from build123d import *

# Parameters (mm, degrees)
BOSS_EXTRUDE1_DEPTH = 12.7
CUT_EXTRUDE2_DEPTH  = 66.991135768
CUT_EXTRUDE1_DEPTH  = 43.597094971
FILLET1_R           = 0.762


with BuildPart() as part:
    # Sketch1 → Boss-Extrude1 (new body)
    with BuildSketch(Plane(origin=(0, 0, 0), x_dir=(1, 0, 0), z_dir=(0, 1, 0))):
        with BuildLine():
            Line((-31.75, -12.7), (31.75, -12.7))
            Line((31.75, -12.7), (31.75, -11.1125))
            Line((31.75, -11.1125), (12.7, -11.1125))
            ThreePointArc((12.7, -11.1125), (8.209871939, -9.252628061), (6.35, -4.7625))
            Line((6.35, -4.7625), (6.35, 4.7625))
            ThreePointArc((6.35, 4.7625), (8.209871939, 9.252628061), (12.7, 11.1125))
            Line((12.7, 11.1125), (31.75, 11.1125))
            Line((31.75, 11.1125), (31.75, 12.7))
            Line((31.75, 12.7), (-31.75, 12.7))
            Line((-31.75, 12.7), (-31.75, 11.1125))
            Line((-31.75, 11.1125), (-12.7, 11.1125))
            ThreePointArc((-12.7, 11.1125), (-8.209871939, 9.252628061), (-6.35, 4.7625))
            Line((-6.35, 4.7625), (-6.35, -4.7625))
            ThreePointArc((-6.35, -4.7625), (-8.209871939, -9.252628061), (-12.7, -11.1125))
            Line((-12.7, -11.1125), (-31.75, -11.1125))
            Line((-31.75, -11.1125), (-31.75, -12.7))
        make_face()
    extrude(amount=BOSS_EXTRUDE1_DEPTH)

    # Sketch3 → Cut-Extrude2 (cut, through all)
    with BuildSketch(Plane.ZY.offset(31.75)):
        Polygon((11.1125, 12.7), (4.7625, 12.7), (-4.7625, 12.7), (-11.1125, 12.7), (-9.525, 6.35), (9.525, 6.35), align=None)
    extrude(amount=-CUT_EXTRUDE2_DEPTH, mode=Mode.SUBTRACT)

    # Sketch2 → Cut-Extrude1 (cut, through all)
    with BuildSketch(Plane.XY.offset(12.7)):
        with BuildLine():
            ThreePointArc((-29.953948776, 4.553948776), (-30.697897552, 6.35), (-29.953948776, 8.146051224))
            Line((-29.953948776, 8.146051224), (-25.4, 12.7))
            Line((-25.4, 12.7), (-31.75, 12.7))
            Line((-31.75, 12.7), (-31.75, 0))
            Line((-31.75, 0), (-25.4, 0))
            Line((-25.4, 0), (-29.953948776, 4.553948776))
        make_face()
        with BuildLine():
            Line((31.75, 12.7), (25.4, 12.7))
            Line((25.4, 12.7), (29.953948776, 8.146051224))
            ThreePointArc((29.953948776, 8.146051224), (30.697897552, 6.35), (29.953948776, 4.553948776))
            Line((29.953948776, 4.553948776), (25.4, 0))
            Line((25.4, 0), (31.75, 0))
            Line((31.75, 0), (31.75, 12.7))
        make_face()
    extrude(amount=-CUT_EXTRUDE1_DEPTH, mode=Mode.SUBTRACT)

    # Sketch4 → Revolve1 (revolve)
    with BuildSketch(Plane.ZY.offset(22.86), mode=Mode.PRIVATE) as revolve1_sk:
        with BuildLine():
            Line((12.7, 6.35), (12.7, 11.43))
            ThreePointArc((12.7, 11.43), (13.881381744, 9.01113492), (14.2875, 6.35))
            Line((14.2875, 6.35), (12.7, 6.35))
        make_face()
    revolve1 = revolve(revolve1_sk.sketch.rotate(Axis((-22.86, 6.35, 0), (0, 0, 1)), 180), axis=Axis((-22.86, 6.35, 0), (0, 0, 1)))

    # Mirror1: Revolve1 across plane
    add(revolve1.mirror(Plane.XY))

    # Sketch5 → Revolve2 (revolve)
    with BuildSketch(Plane(origin=(22.86, 0, 0), x_dir=(0, 0, -1), z_dir=(1, 0, 0))):
        with BuildLine():
            Line((11.1125, 6.35), (11.1125, 11.43))
            ThreePointArc((11.1125, 11.43), (9.931118256, 9.01113492), (9.525, 6.35))
            Line((9.525, 6.35), (11.1125, 6.35))
        make_face()
    revolve2 = revolve(axis=Axis((22.86, 6.35, -9.525), (0, 0, 1)))

    # Mirror2: Revolve2 across plane
    add(revolve2.mirror(Plane.XY))

    # Fillet1
    fillet1_edges = [part.edges().sort_by_distance(p)[0] for p in [
        (-27.676974388, 10.423025612, 11.1125),
        (-25.4, 12.7, 11.90625),
        (-27.676974388, 2.276974388, 12.7),
        (-30.697897552, 6.35, -11.1125),
        (-30.697897552, 6.35, 11.1125),
        (-27.676974388, 2.276974388, -11.1125),
        (-27.676974388, 2.276974388, 11.1125),
        (-30.697897552, 6.35, -12.7),
        (-27.676974388, 2.276974388, -12.7),
        (-27.676974388, 10.423025612, 12.7),
        (30.697897552, 6.35, 12.7),
        (25.4, 12.7, 11.90625),
        (25.4, 12.7, -11.90625),
        (27.676974388, 10.423025612, 12.7),
        (27.676974388, 2.276974388, 11.1125),
        (27.676974388, 2.276974388, -11.1125),
        (27.676974388, 2.276974388, -12.7),
        (30.697897552, 6.35, 11.1125),
        (27.676974388, 10.423025612, 11.1125),
        (27.676974388, 10.423025612, -11.1125),
        (30.697897552, 6.35, -12.7),
        (27.676974388, 10.423025612, -12.7),
        (27.676974388, 2.276974388, 12.7),
        (30.697897552, 6.35, -11.1125),
        (-30.697897552, 6.35, 12.7),
        (-25.4, 12.7, -11.90625),
        (-27.676974388, 10.423025612, -11.1125),
        (-27.676974388, 10.423025612, -12.7),
    ]]
    fillet(fillet1_edges, radius=FILLET1_R)


solid = part.part
CAD build for the part. Positions are in the model's coordinates, mm. A direction names the side the tool comes from. Give positions to 0.01 mm unless a question says otherwise; leave off trailing zeros. Loops run counter-clockwise (first coordinate to the right, second up) from the corner with the lowest first, then second, coordinate; pieces in that order, holes last. Notation, with made-up numbers: M 62.25,38.25 L 84.25,38.25 A22 cw 84.25,70.25 Z; hole C -9,6 d3. An arc over 180 degrees is marked long. One line per question, with ' | ' between items. Start each with the question number.
1. Two-plate mould, pull along Z, no slides. Class faces 5 (the face through (27.21, 2.13, -12.48)), 6 (the face through (0, 12.7, -12)), 7 (the face through (27.22, 10.57, -11.34)): pulls with the +Z half, pulls with the -Z half, needs draft (parallel to the pull), parting line crosses it, or undercut.
2. Flat gauge pins, fed straight in: pin 1 (4 mm diameter, centred on y = 7, z = 6, fed in from -X); pin 2 (1.9 mm diameter, centred on y = 3.5, z = 1.5, fed in from +X); pin 3 (6.5 mm diameter, centred on x = 21, y = 8.5, fed in from +Z). Where does each tip first touch, or does it go through?
3. Saw through at A-A on x = 14. Give the cut face in (y, z).
4. 3-axis set-ups, long thin cutter, end or side, ignore diameter. For faces 1 (the face through (-27.21, 2.13, -11.33)), 2 (the face through (-20, 6, -11.112)), 3 (the face through (-0.178, 9.481, 10.308)), 4 (the face through (27.21, 2.13, 12.48)): which of +Z, -Z, +X, -X, +Y, -Y reach the whole face in a straight line?
5. Saw through at D-D on x = -19. Give the cut face in (y, z).
6. Probe L1, parallel to Z at x = 15.5, y = 1; L2, parallel to Y at x = 2.5, z = -7.25; L3, parallel to Z at x = -10, y = 3.75. List the from-to ranges inside material, lowest first. Write a range as from..to.
7. Saw through at C-C on z = 2.75. Give the cut face in (x, y), plus the area to 3 significant figures.
Result sheet:
1) face 5: pulls with the -Z half | face 6: needs draft | face 7: undercut
2) pin 1: stops at x = -7.17 | pin 2: stops at x = 6.35 | pin 3: stops at z = 12.7
3) outline: M 0,-12.7 L 12.7,-12.7 L 12.7,-11.11 L 0,-11.11 Z; M 0,11.11 L 12.7,11.11 L 12.7,12.7 L 0,12.7 Z
4) face 1: -X, -Y | face 2: -X, +Y, -Y | face 3: -X, +Y | face 4: +Z, +X, -Y
5) outline: M 0,-12.7 L 3.05,-12.7 A8.04 ccw 9.65,-12.7 L 12.7,-12.7 L 12.7,-11.11 L 0,-11.11 Z; M 0,11.11 L 12.7,11.11 L 12.7,12.7 L 9.65,12.7 A8.04 ccw 3.05,12.7 L 0,12.7 Z
6) L1: z = -12.7..-11.11, 11.11..12.7 | L2: y = 0..6.35 | L3: z = -12.7..-10.51, 10.51..12.7
7) outline: M -6.35,0 L 6.35,0 L 6.35,6.35 L -6.35,6.35 Z | area: 80.6 mm^2
